from build123d import *

# Parameters (mm, degrees)
F2_T     = -2
F5_DEPTH = 50


with BuildPart() as f1:
    # F0 (on Top) → F1 (revolve)
    with BuildSketch(Plane.XY):
        Polygon((-25.3351479258, 22.5523764878), (-29.1700512171, 18.1462019682), (18.6146012928, -23.4430542826), (22.4495045841, -19.036879763), align=None)
    revolve(axis=Axis((-5.2777249621, -2.6484261572, 0), (0.754313236, -0.6565146929, 0)))

    # F2
    f2_openings = [f1.faces().sort_by_distance(p)[0] for p in [
        (-29.170051, 18.146202, 0),
        (18.614601, -23.443054, 0),
    ]]
    offset(amount=F2_T, openings=f2_openings)

    # F4 (on offset) → F5 (intersect)
    with BuildSketch(Plane.XY.offset(25)):
        Polygon((-17.0640610158, -8.8143590838), (-10.2202640846, -15.1658570394), (26.4985691756, -15.1658570394), (26.4985691756, 0), (0, 0), (5.9569892474, 13.9789059758), (-9.5655685291, 19.4225348532), align=None)
    extrude(amount=-F5_DEPTH, mode=Mode.INTERSECT)


solid = f1.part
The listing builds one solid part. Answer for the finished solid, in the listing's coordinates (mm). Coordinates: 2 decimals unless noted, no trailing zeros. Order: outer loops, then holes, each group sorted by start corner. A loop starts at its lowest first (then second) coordinate and runs counter-clockwise, first axis right, second up. Notation, with made-up numbers: (-14.75, 36) -> (2.25, 36) arc R21 cw to (2.25, 69) -> close; hole circle Ø5 at (81.5, 5.25). An arc over 180 degrees is marked (long way). Answer in a Markdown table with one row per item. Add a question column.
Item 1: Determine the mould class of faces 1 (the face through (-13.87, 3.22, -3.81)), 2 (the face through (9, -15.166, 4)), 3 (the face through (0.96, -3.22, 1.15)) for opening direction X: +X half, -X half, draft (parallel to the pull), parting line (faces both ways), or undercut.
Item 2: Each of these flat-tipped pins is pushed along its axis until it touches: P1, Ø1.5, axis at y = -9, z = 3, coming from the -X side; P2, Ø5, axis at x = 11.5, y = -9.5, coming from the +Z side; P3, Ø2, axis at y = 0.5, z = 0, coming from the -X side. Where does it stop, or does it pass through?
Item 3: Find section A-A (z = -3.25). Write down the section's boundary in (x, y).
Item 4: Find the intervals of material crossed by L1, parallel to Y at x = -6.5, z = -1; L2, parallel to Y at x = -1.5, z = -3; L3, parallel to X at y = -9.5, z = 1.75, in increasing order. Write a range as from..to.
Item 5: Find section B-B (z = 0.5). Write down the section's boundary in (x, y), then the cut area to 3 significant figures.
Result set:
| question | item | result |
|---|---|---|
| 1 | face 1 | -X half |
| 1 | face 2 | draft |
| 1 | face 3 | undercut |
| 2 | P1 | stops at x = -6.68 |
| 2 | P2 | stops at z = 4.79 |
| 2 | P3 | stops at x = -14.86 |
| 3 | outline | (-14.91, -0.7) -> (1.71, -15.17) -> (5.99, -15.17) -> (-14.11, 2.32) -> close; (-12.94, 6.73) -> (12.22, -15.17) -> (16.5, -15.17) -> (-12.13, 9.75) -> close |
| 4 | L1 | y = -9.21..-6.5, 3.33..6.04 |
| 4 | L2 | y = -12.58..-9.12, -2.76..0.71 |
| 4 | L3 | x = -5.89..-2.61, 7.8..11.08 |
| 5 | outline | (-15.19, -1.74) -> (0.24, -15.17) -> (3.3, -15.17) -> (-14.61, 0.43) -> close; (-12.43, 8.63) -> (14.91, -15.17) -> (17.97, -15.17) -> (0.54, 0) -> (0, 0) -> (0.15, 0.35) -> (-11.86, 10.79) -> close |
| 5 | area | 121 mm² |
